Geometry: see drawing. Coordinates: mm, zero at the bounding-box minimum. Give positions to 0.01 mm unless a question says otherwise; leave off trailing zeros. Loops run counter-clockwise (first coordinate to the right, second up) from the corner with the lowest first, then second, coordinate; pieces in that order, holes last. Notation, with made-up numbers: (2.25, 47.25) -> (7.25, 47.25) arc R37 cw to (7.25, 86.25) -> close; hole circle Ø2 at (-31.5, -34.75). An arc over 180 degrees is marked (long way). Return JSON: item names as keys, results as strings. Group by question number.
(1) Pin query (flat end, axial travel): pin 1 (1 mm diameter, centred on x = 43, z = 2.5, fed in from -Y); pin 2 (2 mm diameter, centred on x = 9.5, y = 93.5, fed in from -Z). Return the tip coordinate at first contact, or that it passes through.
(2) Cut plane A-A on x = 9.5. Return loops of the section in (y, z), then the cut area to 3 significant figures.
(3) Ray query, line 1 (Y direction, x = 93.5, z = 2.1); line 2 (Y direction, x = 9, z = 1.3). Return the intervals inside material, ascending. Write a range as from..to.
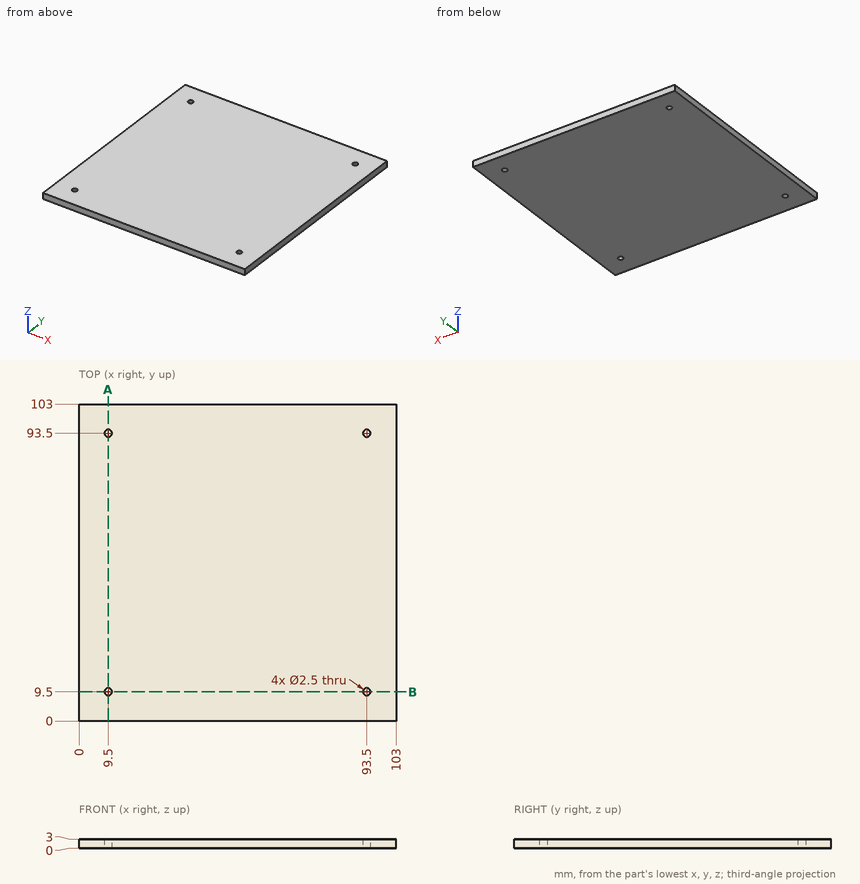
Answers:
{
 "1": {"pin 1": "y = 0", "pin 2": "through"},
 "2": {"outline": "(0, 0) -> (8.25, 0) -> (8.25, 3) -> (0, 3) -> close; (10.75, 0) -> (92.25, 0) -> (92.25, 3) -> (10.75, 3) -> close; (94.75, 0) -> (103, 0) -> (103, 3) -> (94.75, 3) -> close", "area": "294 mm²"},
 "3": {"line 1": "0..8.25, 10.75..92.25, 94.75..103", "line 2": "0..8.35, 10.65..92.35, 94.65..103"}
}
